Source: CAD feature listing. Evaluate the final solid. Frame: model axes, mm. A direction names the side the tool comes from. Coordinates: 2 decimals unless noted, no trailing zeros. Order: outer loops, then holes, each group sorted by start corner. A loop starts at its lowest first (then second) coordinate and runs counter-clockwise, first axis right, second up.
Item 1: Reachability of faces 4 (the flat face through (-14, 0, 43)), 5 (the flat face through (-56.25, 2, -15)), 6 (the flat face through (61, 2, 2.5)) from +Z, -Z, +X, -X, +Y, -Y: full face, straight path, thin tool, end or side. Return the list, or none.
Item 2: Contact query for flat-ended pins moving along their axis: P1, Ø1.4, axis at y = 2.5, z = -19.5, coming from the -X side; P2, Ø5, axis at x = -54.95, z = 9.5, coming from the -Y side; P3, Ø1.4, axis at y = 2, z = -12, coming from the +X side; P4, Ø2.5, axis at x = 0, z = 57.5, coming from the +Y side. Output: stop coordinate, or through.
Item 3: Ray query, line 1 (X direction, y = 3.4, z = 9.5); line 2 (X direction, y = 2.9, z = 57.5); line 3 (X direction, y = 2.65, z = -22.5). Return the intervals inside material, ascending.
Item 4: Section D-D on y = 3.2. State how many separate pieces and enclosed holes the cut face has, then the cut area to 3 significant figures.
Item 5: Section A-A on x = -32. Return the cut outline in (y, z), then the cut area to 3 significant figures.
Item 6: Mould query, pull axis Z, two halves, no side actions, for faces 1 (the cylindrical face through (56.44, 2.34, 9.7)), 2 (the flat face through (56.25, 2, -15)), 3 (the cylindrical face through (-1.394, 2.342, 64.985)). Classes: released by +Z, released by -Z, zero draft, split by the parting line, or undercut.
Item 7: Section B-B on z = 0. Return the cut outline in (x, y).
Item 8: Section C-C on x = 0. Return the cut outline in (y, z), then the cut area to 4 significant figures.
from build123d import *

# Parameters (mm, degrees)
SKETCH1_R           = 65
SKETCH1_R_2         = 1.5
SKETCH1_R_3         = 45
BOSS_EXTRUDE1_DEPTH = 4.75
SKETCH3_W           = 10
SKETCH3_H           = 5
CUT_EXTRUDE1_DEPTH  = 5
CUT_EXTRUDE2_DEPTH  = 93.012567076
SKETCH5_R           = 1.5
CUT_EXTRUDE3_DEPTH  = 93.012567076


with BuildPart() as part:
    # Sketch1 → Boss-Extrude1 (new body)
    with BuildSketch(Plane(origin=(0, 0, 0), x_dir=(1, 0, 0), z_dir=(0, 1, 0))):
        with Locations(Location((0, 0, 0), (0, 0, 270))):
            Circle(SKETCH1_R)
        with Locations(Location((0, -57.5, 0), (0, 0, 270))):
            Circle(SKETCH1_R_2, mode=Mode.SUBTRACT)
        with Locations(Location((40.658639918, -40.658639918, 0), (0, 0, 270))):
            Circle(SKETCH1_R_2, mode=Mode.SUBTRACT)
        with Locations(Location((40.658639918, 40.658639918, 0), (0, 0, 270))):
            Circle(SKETCH1_R_2, mode=Mode.SUBTRACT)
        with Locations(Location((0, 57.5, 0), (0, 0, 90))):
            Circle(SKETCH1_R_2, mode=Mode.SUBTRACT)
        with Locations(Location((-40.658639918, 40.658639918, 0), (0, 0, 90))):
            Circle(SKETCH1_R_2, mode=Mode.SUBTRACT)
        with Locations(Location((-40.658639918, -40.658639918, 0), (0, 0, 90))):
            Circle(SKETCH1_R_2, mode=Mode.SUBTRACT)
        with Locations(Location((0, 0, 0), (0, 0, 270))):
            Circle(SKETCH1_R_3, mode=Mode.SUBTRACT)
    extrude(amount=BOSS_EXTRUDE1_DEPTH)

    # Sketch3 → Cut-Extrude1 (cut)
    with BuildSketch(Plane(origin=(0, 4.75, 0), x_dir=(1, 0, 0), z_dir=(0, 1, 0))):
        with Locations((61.25, 0)):
            Rectangle(SKETCH3_W, SKETCH3_H)
        with Locations((-61.25, 0)):
            Rectangle(SKETCH3_W, SKETCH3_H)
    extrude(amount=-CUT_EXTRUDE1_DEPTH, mode=Mode.SUBTRACT)

    # Sketch4 → Cut-Extrude2 (cut, through all)
    with BuildSketch(Plane(origin=(0, 4.75, 0), x_dir=(1, 0, 0), z_dir=(0, 1, 0))):
        with BuildLine():
            Line((-64.951905284, 2.5), (-56.25, 2.5))
            Line((-56.25, 2.5), (-56.25, 32.572035552))
            ThreePointArc((-56.25, 32.572035552), (-62.438428004, 18.067725599), (-64.951905284, 2.5))
        make_face()
        with BuildLine():
            ThreePointArc((64.951905284, 2.5), (62.438428004, 18.067725599), (56.25, 32.572035552))
            Line((56.25, 32.572035552), (56.25, 2.5))
            Line((56.25, 2.5), (64.951905284, 2.5))
        make_face()
    extrude(amount=-CUT_EXTRUDE2_DEPTH, mode=Mode.SUBTRACT)

    # Sketch5 → Cut-Extrude3 (cut, through all)
    with BuildSketch(Plane.XZ):
        with Locations(Location((54.951905284, 9.5, 0), (0, 0, 270))):
            Circle(SKETCH5_R)
        with Locations(Location((-54.951905284, 9.5, 0), (0, 0, 90))):
            Circle(SKETCH5_R)
    extrude(amount=-CUT_EXTRUDE3_DEPTH, mode=Mode.SUBTRACT)


solid = part.part
Answer list:
1. face 4: +Z, -Z, +X, -X, -Y
1. face 5: -Z, -X, +Y, -Y
1. face 6: -Z, +X, +Y, -Y
2. P1: stops at x = -56.25
2. P2: stops at y = 0
2. P3: stops at x = 56.25
2. P4: passes through
3. line 1: x = -64.3 to -56.45, -53.45 to -43.99, 43.99 to 53.45, 56.45 to 64.3
3. line 2: x = -30.31 to -1.5, 1.5 to 30.31
3. line 3: x = -56.25 to -38.97, 38.97 to 56.25
4. separate pieces: 1
4. enclosed holes: 9
4. area: 6,430 mm2
5. outline: (0, -56.58) - (4.75, -56.58) - (4.75, -31.64) - (0, -31.64) - close; (0, 31.64) - (4.75, 31.64) - (4.75, 56.58) - (0, 56.58) - close
5. area: 237 mm2
6. face 1: undercut
6. face 2: zero draft
6. face 3: released by +Z
7. outline: (-56.25, 0) - (-45, 0) - (-45, 4.75) - (-56.25, 4.75) - close; (45, 0) - (56.25, 0) - (56.25, 4.75) - (45, 4.75) - close
8. outline: (0, -65) - (4.75, -65) - (4.75, -59) - (0, -59) - close; (0, -56) - (4.75, -56) - (4.75, -45) - (0, -45) - close; (0, 45) - (4.75, 45) - (4.75, 56) - (0, 56) - close; (0, 59) - (4.75, 59) - (4.75, 65) - (0, 65) - close
8. area: 161.5 mm2
